Check sheet for the drawn part. Datum: minimum x, y, z corner. Units: mm. A direction names the side the tool comes from. Round coordinates to 2 decimals unless told otherwise and drop trailing zeros. Write each loop counter-clockwise with the first axis right and the second up, starting at its lowest first coordinate (ties: lowest second). Pieces come first, ordered by that corner, then holes. Notation, with made-up numbers: (2, 61.5) - (34, 61.5) arc R15 ccw to (34, 72.5) - close; hole circle Ø5 at (-10.5, -26.75). An arc over 180 degrees is marked (long way). Answer as a JSON object with one key per item and string values.
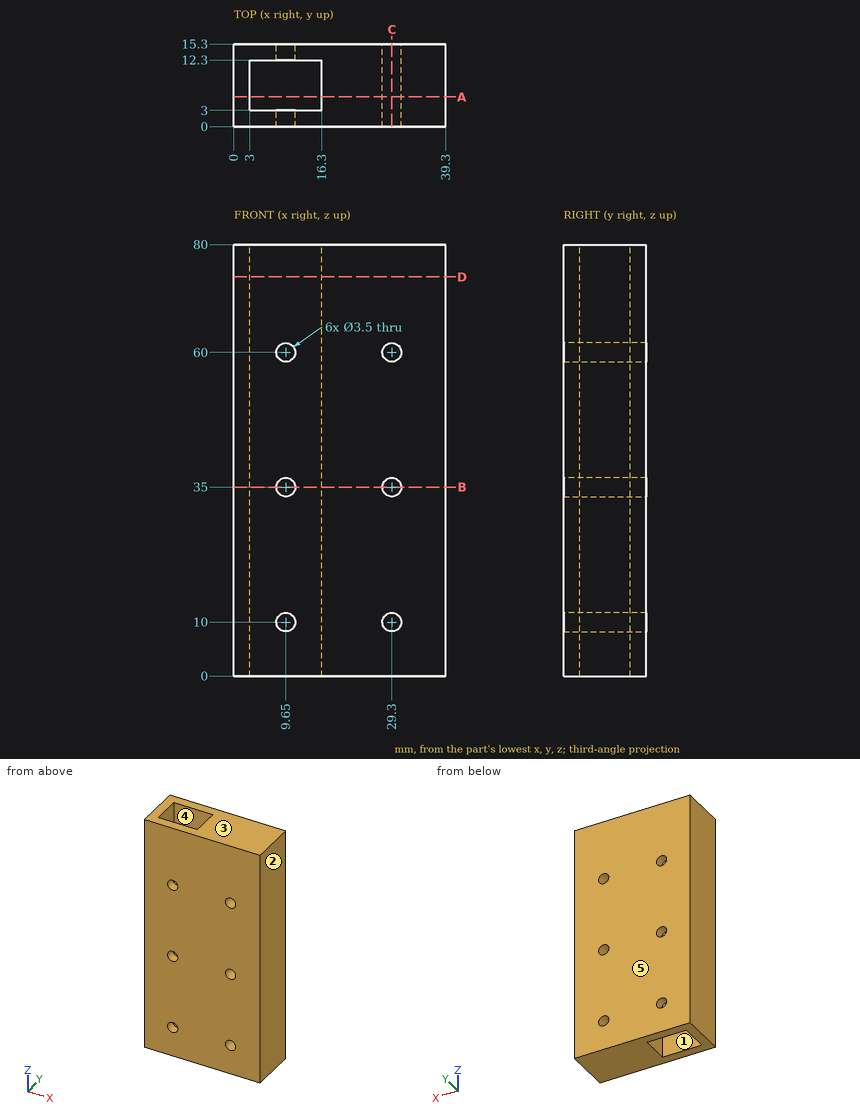
1. Go/stop test with a flat-tipped pin: pin 1 (2 mm diameter, centred on x = 30, y = 6, fed in from -Z). Record where the tip stops, or that it passes through.
Completed:
{"pin 1": "stops at z = 0"}
2. Cross-section at C-C (x = 29.3). Record the boundary of the cut face in (y, z).
Completed:
{"outline": "(0, 0) - (15.3, 0) - (15.3, 8.25) - (0, 8.25) - close; (0, 11.75) - (15.3, 11.75) - (15.3, 33.25) - (0, 33.25) - close; (0, 36.75) - (15.3, 36.75) - (15.3, 58.25) - (0, 58.25) - close; (0, 61.75) - (15.3, 61.75) - (15.3, 80) - (0, 80) - close"}
3. Material ranges on probe 1 along X at (y, z) = (5.5, 35); probe 2 along X at (y, z) = (13.3, 60); probe 3 along Y at (x, z) = (7.5, 50), recorded low to high. Write a range as from..to.
Completed:
{"probe 1": "x = 0..3, 16.3..27.55, 31.05..39.3", "probe 2": "x = 0..7.9, 11.4..27.55, 31.05..39.3", "probe 3": "y = 0..3, 12.3..15.3"}
4. Mould release check, pull along X, two halves, no side actions. Record for the marked faces 1, 2 and 3: released by +X, released by -X, zero draft, split by the parting line, or undercut.
Completed:
{"face 1": "undercut", "face 2": "released by +X", "face 3": "zero draft"}
5. Cross-section at D-D (z = 74). Record the boundary of the cut face in (x, y).
Completed:
{"outline": "(0, 0) - (39.3, 0) - (39.3, 15.3) - (0, 15.3) - close; hole (3, 3) - (16.3, 3) - (16.3, 12.3) - (3, 12.3) - close"}
6. Access from +Z, -Z, +X, -X, +Y, -Y to the whole of each face (thin tool, end or side, straight path). Record for the marked faces 4 and 5.
Completed:
{"face 4": "+Z, -Z", "face 5": "+Z, -Z, +X, -X, +Y"}
7. Cross-section at A-A (y = 5.5). Record the boundary of the cut face in (x, z), plus the area to 3 significant figures.
Completed:
{"outline": "(0, 0) - (3, 0) - (3, 80) - (0, 80) - close; (16.3, 0) - (39.3, 0) - (39.3, 80) - (16.3, 80) - close; hole circle Ø3.5 at (29.3, 10); hole circle Ø3.5 at (29.3, 35); hole circle Ø3.5 at (29.3, 60)", "area": "2,050 mm^2"}
8. Cross-section at B-B (z = 35). Record the boundary of the cut face in (x, y).
Completed:
{"outline": "(0, 0) - (7.9, 0) - (7.9, 3) - (3, 3) - (3, 12.3) - (7.9, 12.3) - (7.9, 15.3) - (0, 15.3) - close; (11.4, 0) - (27.55, 0) - (27.55, 15.3) - (11.4, 15.3) - (11.4, 12.3) - (16.3, 12.3) - (16.3, 3) - (11.4, 3) - close; (31.05, 0) - (39.3, 0) - (39.3, 15.3) - (31.05, 15.3) - close"}
